Geometry: see drawing. Coordinates: mm, zero at the bounding-box minimum. Coordinates: 2 decimals unless noted, no trailing zeros. Use a Markdown table: item, result. Add a question column.
1. Ray query, L1, parallel to Y at x = 39, z = 39; L2, parallel to Y at x = 31.75, z = 24.5 (1 decimal); L3, parallel to X at y = 18.5, z = 39 (1 decimal). Return the intervals inside material, ascending. Write a range as [from, to].
2. Draft query along Y for the marked faces 1, 2 and 3. Return one class per face: released by +Y, released by -Y, zero draft, split by the parting line, or undercut.
3. Contact query for flat-ended pins moving along their axis: P1, Ø1.5, axis at y = 26.5, z = 29, coming from the +X side; P2, Ø0.8, axis at x = 32, y = 18.5, coming from the -Z side; P3, Ø1, axis at x = 10, z = 9.5, coming from the -Y side. Output: stop coordinate, or through.
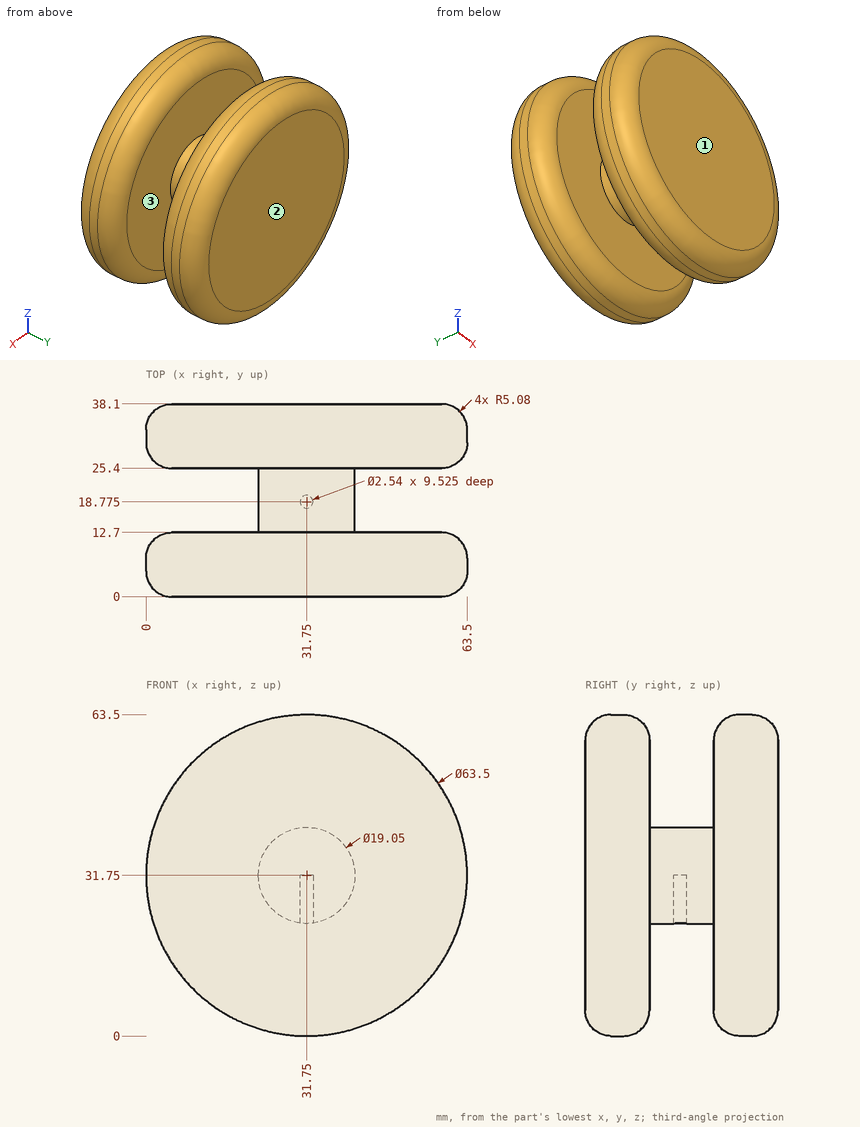
Resolved:
| question | item | result |
|---|---|---|
| 1 | L1 | [0, 12.7], [25.4, 38.1] |
| 1 | L2 | [0, 17.5], [20, 38.1] |
| 1 | L3 | [25.6, 37.9] |
| 2 | face 1 | released by -Y |
| 2 | face 2 | released by +Y |
| 2 | face 3 | undercut |
| 3 | P1 | x = 62.22 |
| 3 | P2 | z = 31.75 |
| 3 | P3 | y = 1.88 |
